CAD build for the part. Positions are in the model's coordinates, mm. Face numbers are marked on the shaded views. A direction names the side the tool comes from. Give positions to 0.01 mm unless a question says otherwise; leave off trailing zeros. Write each loop counter-clockwise with the first axis right and the second up, starting at its lowest first coordinate (ties: lowest second). Pieces come first, ordered by that corner, then holes. Notation, with made-up numbers: (8, -40) - (60, -40) arc R17 cw to (60, -26) - close; hole circle Ø11 at (78, 64.25). An arc over 180 degrees is marked (long way). Answer as a JSON object with one key per item and string values.
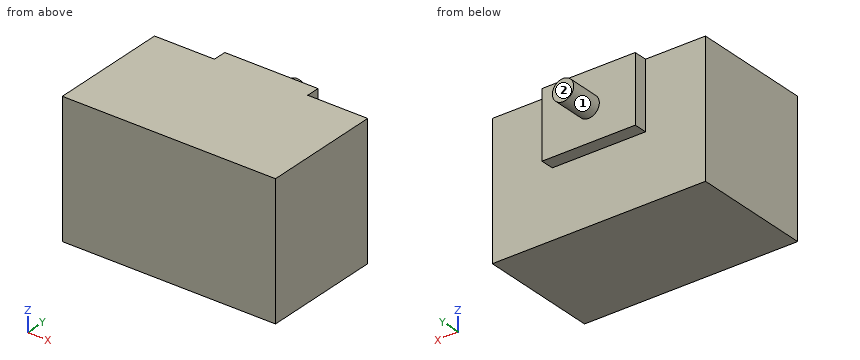
from build123d import *

# Parameters (mm, degrees)
SKETCH_1_W      = 1600
SKETCH_1_H      = 1000
EXTRUDE_1_DEPTH = 900
SKETCH_2_W      = 700
SKETCH_2_H      = 500
EXTRUDE_2_DEPTH = 100
SKETCH_5_R      = 80
EXTRUDE_5_DEPTH = 250


with BuildPart() as part:
    # 草图1 → 凸台-拉伸1 (new body)
    with BuildSketch(Plane(origin=(0, 0, 0), x_dir=(1, 0, 0), z_dir=(0, 1, 0))):
        Rectangle(SKETCH_1_W, SKETCH_1_H)
    extrude(amount=EXTRUDE_1_DEPTH)

    # 草图2 → 凸台-拉伸2 (add)
    with BuildSketch(Plane(origin=(0, 900, 0), x_dir=(1, 0, 0), z_dir=(0, 1, 0))):
        with Locations((0, -250)):
            Rectangle(SKETCH_2_W, SKETCH_2_H)
    extrude(amount=EXTRUDE_2_DEPTH)

    # 草图5 → 凸台-拉伸5 (add)
    with BuildSketch(Plane(origin=(0, 1000, 0), x_dir=(1, 0, 0), z_dir=(0, 1, 0))):
        with Locations((0, -250)):
            Circle(SKETCH_5_R)
    extrude(amount=EXTRUDE_5_DEPTH)


solid = part.part
(1) 3-axis set-ups, long thin cutter, end or side, ignore diameter. For the marked faces 1 and 2: which of +Z, -Z, +X, -X, +Y, -Y reach the whole face in a straight line?
Answer key:
{"face 1": "+Y", "face 2": "+Z, -Z, +X, -X, +Y"}
(2) Saw through at C-C, the plane y = 924.5. Give the cut face in (x, z), and give its area (3 significant figures).
Answer key:
{"outline": "(-350, 0) - (350, 0) - (350, 500) - (-350, 500) - close", "area": "350,000 mm²"}
(3) Saw through at A-A, the plane z = 250. Give the cut face in (x, y).
Answer key:
{"outline": "(-800, 0) - (800, 0) - (800, 900) - (350, 900) - (350, 1000) - (80, 1000) - (80, 1250) - (-80, 1250) - (-80, 1000) - (-350, 1000) - (-350, 900) - (-800, 900) - close"}
(4) Probe L1, parallel to Y at x = -37.5, z = 325.5; L2, parallel to Y at x = -27, z = -88; L3, parallel to X at y = 1111, z = 182. List the from-to ranges inside material, lowest first. Write a range as [from, to].
Answer key:
{"L1": "y = [0, 1000]", "L2": "y = [0, 900]", "L3": "x = [-42.14, 42.14]"}
(5) Saw through at B-B, the plane x = 0. Give the cut face in (y, z), and give its area (3 significant figures).
Answer key:
{"outline": "(0, -500) - (900, -500) - (900, 0) - (1000, 0) - (1000, 170) - (1250, 170) - (1250, 330) - (1000, 330) - (1000, 500) - (0, 500) - close", "area": "990,000 mm²"}
(6) Saw through at D-D, the plane x = -293. Give the cut face in (y, z).
Answer key:
{"outline": "(0, -500) - (900, -500) - (900, 0) - (1000, 0) - (1000, 500) - (0, 500) - close"}
